For this review, take the finished solid that the model builds, in its own axes (mm). Give positions to 0.01 mm unless a question says otherwise; leave off trailing zeros. Order: outer loops, then holes, each group sorted by start corner. A loop starts at its lowest first (then second) coordinate and runs counter-clockwise, first axis right, second up. Notation, with made-up numbers: (-29.5, 46) - (-12.5, 46) arc R27 ccw to (-12.5, 64) - close; hole circle Ø3 at (3.25, -16). An arc over 180 degrees is marked (long way). One line per item, written item: value.
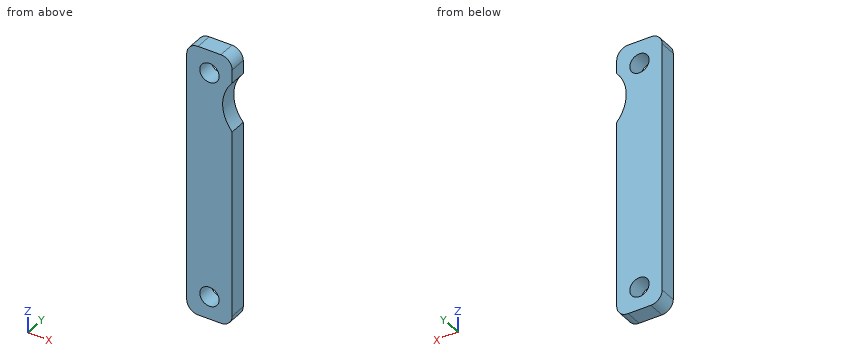
```python
from build123d import *

# Parameters (mm, degrees)
SKETCH_1_R          = 1.7
EXTRUDE_1_DEPTH     = 3
CUT_EXTRUDE_1_DEPTH = 3


with BuildPart() as part:
    # 草圖1 → 填料-伸長1 (new body)
    with BuildSketch(Plane(origin=(0, 0, 0), x_dir=(1, 0, 0), z_dir=(0, 1, 0))):
        with BuildLine():
            Line((-2, 24), (2, 24))
            ThreePointArc((2, 24), (3.414213562, 23.414213562), (4, 22))
            Line((4, 22), (4, -22))
            ThreePointArc((4, -22), (3.414213562, -23.414213562), (2, -24))
            Line((2, -24), (-2, -24))
            ThreePointArc((-2, -24), (-3.414213562, -23.414213562), (-4, -22))
            Line((-4, -22), (-4, 22))
            ThreePointArc((-4, 22), (-3.414213562, 23.414213562), (-2, 24))
        make_face()
        with Locations(Location((0, 20, 0), (0, 0, 270))):
            Circle(SKETCH_1_R, mode=Mode.SUBTRACT)
        with Locations(Location((0, -20, 0), (0, 0, 90))):
            Circle(SKETCH_1_R, mode=Mode.SUBTRACT)
    extrude(amount=EXTRUDE_1_DEPTH)

    # 草圖2 → 除料-伸長1 (cut)
    with BuildSketch(Plane(origin=(0, 3, 0), x_dir=(1, 0, 0), z_dir=(0, 1, 0))):
        with BuildLine():
            Line((4, -10.936925409), (8.605915435, -21.790363308))
            ThreePointArc((8.605915435, -21.790363308), (2.8399706, -17.8332456), (4, -10.936925409))
        make_face()
    extrude(amount=-CUT_EXTRUDE_1_DEPTH, mode=Mode.SUBTRACT)


solid = part.part
```
(1) Take a section at A-A (x = 0). Write out the cut boundary in (y, z).
Answers below:
outline: (0, -24) - (3, -24) - (3, -21.7) - (0, -21.7) - close; (0, -18.3) - (3, -18.3) - (3, 18.3) - (0, 18.3) - close; (0, 21.7) - (3, 21.7) - (3, 24) - (0, 24) - close
(2) Wall thickness on line 1 (Z direction, x = 1.5, y = 2.1); line 2 (Z direction, x = -1, y = 0.95); line 3 (X direction, y = 0.95, z = 20): over which ranges is each line inside the solid? List them lowest first. Write a range as from..to.
Answers below:
line 1: z = -24..-20.8, -19.2..19.2, 20.8..24
line 2: z = -24..-21.37, -18.63..18.63, 21.37..24
line 3: x = -4..-1.7, 1.7..4
(3) Take a section at C-C (y = 2.45). Write out the cut boundary in (x, z).
Answers below:
outline: (-4, -22) arc R2 ccw to (-2, -24) - (2, -24) arc R2 ccw to (4, -22) - (4, 10.94) arc R6.5 cw to (4, 19.65) - (4, 22) arc R2 ccw to (2, 24) - (-2, 24) arc R2 ccw to (-4, 22) - close; hole circle Ø3.4 at (0, -20); hole circle Ø3.4 at (0, 20)
(4) Take a section at D-D (x = 3.5). Write out the cut boundary in (y, z).
Answers below:
outline: (0, -23.32) - (3, -23.32) - (3, 11.56) - (0, 11.56) - close; (0, 19.02) - (3, 19.02) - (3, 23.32) - (0, 23.32) - close
(5) Take a section at B-B (z = -20). Write out the cut boundary in (x, y), then the cut area to 3 significant figures.
Answers below:
outline: (-4, 0) - (-1.7, 0) - (-1.7, 3) - (-4, 3) - close; (1.7, 0) - (4, 0) - (4, 3) - (1.7, 3) - close
area: 13.8 mm^2
